from build123d import *

# Parameters (mm, degrees)
SKETCH1_W                = 50
SKETCH1_H                = 25
SKETCH1_R                = 1.3
SKETCH1_R_2              = 4.5
BOSS_EXTRUDE1_DEPTH      = 2.5
SKETCH2_W                = 50
SKETCH2_H                = 12
BOSS_EXTRUDE2_DEPTH      = 3
SKETCH3_W                = 50
SKETCH3_H                = 28
BOSS_EXTRUDE3_DEPTH      = 3
SKETCH4_R                = 1.3
CUT_EXTRUDE1_DEPTH       = 16
SKETCH5_W                = 53
SKETCH5_H                = 32.5
SKETCH5_R                = 1.6
SKETCH5_W_2              = 42
SKETCH5_H_2              = 21.5
BOSS_EXTRUDE4_DEPTH      = 4
SKETCH7_R                = 8
CUT_EXTRUDE2_DEPTH       = 5
SKETCH8_W                = 24.55
SKETCH8_H                = 21.5
CUT_EXTRUDE3_DEPTH       = 3.8
BOSS_EXTRUDE6_DEPTH      = 22.95
BOSS_EXTRUDE7_DEPTH      = 2
SKETCH11_R               = 1.6
CUT_EXTRUDE4_DEPTH       = 1.2
SKETCH12_W               = 7
SKETCH12_H               = 21
SKETCH12_R               = 1.6
BOSS_EXTRUDE8_DEPTH      = 7.8
SKETCH13_W               = 0.7
SKETCH13_H               = 5
SKETCH13_H_2             = 4
CUT_EXTRUDE5_DEPTH       = 51
CUT_EXTRUDE5_DEPTH_BACK  = 25.95
SKETCH14_W               = 3
SKETCH14_H               = 4
SKETCH14_W_2             = 25
SKETCH14_H_2             = 5
CUT_EXTRUDE6_DEPTH       = 1
CUT_EXTRUDE6_DEPTH_BACK  = 75.95
SKETCH15_W               = 24.95
SKETCH15_H               = 3
CUT_EXTRUDE7_DEPTH       = 11
CUT_EXTRUDE7_DEPTH_BACK  = 6
SKETCH16_R               = 1.45
SKETCH16_W               = 6
SKETCH16_H               = 5.2
CUT_EXTRUDE8_DEPTH       = 1
CUT_EXTRUDE8_DEPTH_BACK  = 29
SKETCH18_R               = 1.5
CUT_EXTRUDE9_DEPTH       = 1
CUT_EXTRUDE9_DEPTH_BACK  = 16
SKETCH19_R               = 1.3
BOSS_EXTRUDE9_DEPTH      = 3
SKETCH20_R               = 1.5
CUT_EXTRUDE10_DEPTH      = 1
CUT_EXTRUDE10_DEPTH_BACK = 16


with BuildPart() as part:
    # Sketch1 → Boss-Extrude1 (new body, symmetric)
    with BuildSketch(Plane(origin=(0, 0, 0), x_dir=(1, 0, 0), z_dir=(0, 1, 0))):
        Rectangle(SKETCH1_W, SKETCH1_H)
        with Locations((-11.25, 0)):
            Circle(SKETCH1_R, mode=Mode.SUBTRACT)
        with Locations((11.25, 0)):
            Circle(SKETCH1_R_2, mode=Mode.SUBTRACT)
    extrude(amount=BOSS_EXTRUDE1_DEPTH, both=True)

    # Sketch2 → Boss-Extrude2 (add)
    with BuildSketch(Plane.XY.offset(12.5)):
        with Locations((0, 3.5)):
            Rectangle(SKETCH2_W, SKETCH2_H)
    extrude(amount=BOSS_EXTRUDE2_DEPTH)

    # Sketch3 → Boss-Extrude3 (add)
    with BuildSketch(Plane(origin=(0, 9.5, 0), x_dir=(1, 0, 0), z_dir=(0, 1, 0))):
        with Locations((0, -1.5)):
            Rectangle(SKETCH3_W, SKETCH3_H)
    extrude(amount=BOSS_EXTRUDE3_DEPTH)

    # Sketch4 → Cut-Extrude1 (cut, through all)
    with BuildSketch(Plane(origin=(0, 12.5, 0), x_dir=(1, 0, 0), z_dir=(0, 1, 0))):
        with Locations((11.25, 0)):
            Circle(SKETCH4_R)
        with Locations((-11.25, 0)):
            Circle(SKETCH4_R)
    extrude(amount=-CUT_EXTRUDE1_DEPTH, mode=Mode.SUBTRACT)

    # Sketch5 → Boss-Extrude4 (add)
    with BuildSketch(Plane.XZ.offset(2.5)):
        with Locations((21.45, -0.05)):
            Rectangle(SKETCH5_W, SKETCH5_H)
        with Locations((45.75, -5)):
            Circle(SKETCH5_R, mode=Mode.SUBTRACT)
        with Locations((45.75, 4.9)):
            Circle(SKETCH5_R, mode=Mode.SUBTRACT)
        with Locations((-2.85, 4.9)):
            Circle(SKETCH5_R, mode=Mode.SUBTRACT)
        with Locations((-2.85, -5)):
            Circle(SKETCH5_R, mode=Mode.SUBTRACT)
        with Locations((21.45, -0.05)):
            Rectangle(SKETCH5_W_2, SKETCH5_H_2, mode=Mode.SUBTRACT)
    extrude(amount=BOSS_EXTRUDE4_DEPTH)

    # Sketch7 → Cut-Extrude2 (cut)
    with BuildSketch(Plane.XZ.offset(2.5)):
        with Locations((11.25, 0)):
            Circle(SKETCH7_R)
    extrude(amount=-CUT_EXTRUDE2_DEPTH, mode=Mode.SUBTRACT)

    # Sketch8 → Cut-Extrude3 (cut)
    with BuildSketch(Plane.XZ.offset(2.5)):
        with Locations((12.725, -0.05)):
            Rectangle(SKETCH8_W, SKETCH8_H)
    extrude(amount=-CUT_EXTRUDE3_DEPTH, mode=Mode.SUBTRACT)

    # Sketch9 → Boss-Extrude6 (add)
    with BuildSketch(Plane(origin=(25, 0, 0), x_dir=(0, 0, -1), z_dir=(1, 0, 0))):
        Polygon((12.5, 2.5), (-16.2, 2.5), (-16.2, -2.5), (-10.7, -2.5), (-10.7, 1.3), (10.8, 1.3), (10.8, -2.5), (12.5, -2.5), align=None)
    extrude(amount=BOSS_EXTRUDE6_DEPTH)

    # Sketch10 → Boss-Extrude7 (add)
    with BuildSketch(Plane(origin=(47.95, 0, 0), x_dir=(0, 0, -1), z_dir=(1, 0, 0))):
        Polygon((16.3, -2.5), (12.5, -2.5), (12.5, 2.5), (-16.2, 2.5), (-16.2, -6.5), (16.3, -6.5), align=None)
    extrude(amount=BOSS_EXTRUDE7_DEPTH)

    # Sketch11 → Cut-Extrude4 (cut)
    with BuildSketch(Plane.XZ.offset(-1.3)):
        with Locations((-2.85, 4.9)):
            Circle(SKETCH11_R)
        with Locations((-2.85, -5)):
            Circle(SKETCH11_R)
        with Locations((45.75, 4.9)):
            Circle(SKETCH11_R)
        with Locations((45.75, -5)):
            Circle(SKETCH11_R)
    extrude(amount=-CUT_EXTRUDE4_DEPTH, mode=Mode.SUBTRACT)

    # Sketch12 → Boss-Extrude8 (add)
    with BuildSketch(Plane.XZ.offset(-1.3)):
        with Locations((46.45, 0.2)):
            Rectangle(SKETCH12_W, SKETCH12_H)
        with Locations((45.75, 4.9)):
            Circle(SKETCH12_R, mode=Mode.SUBTRACT)
        with Locations((45.75, -5)):
            Circle(SKETCH12_R, mode=Mode.SUBTRACT)
    extrude(amount=BOSS_EXTRUDE8_DEPTH)

    # Sketch13 → Cut-Extrude5 (cut, two sides)
    with BuildSketch(Plane.ZY.offset(-25)) as cut_extrude5_sk:
        with Locations((15.85, 0)):
            Rectangle(SKETCH13_W, SKETCH13_H)
        with Locations((15.85, -4.5)):
            Rectangle(SKETCH13_W, SKETCH13_H_2)
    extrude(amount=CUT_EXTRUDE5_DEPTH, mode=Mode.SUBTRACT)
    extrude(cut_extrude5_sk.sketch, amount=-CUT_EXTRUDE5_DEPTH_BACK, mode=Mode.SUBTRACT)

    # Sketch14 → Cut-Extrude6 (cut, two sides)
    with BuildSketch(Plane.ZY.offset(25)) as cut_extrude6_sk:
        with Locations((14, -4.5)):
            Rectangle(SKETCH14_W, SKETCH14_H)
        Polygon((-16.3, 2.5), (-16.3, -6.5), (12.5, -6.5), (12.5, -2.5), (-12.5, -2.5), (-12.5, 2.5), align=None)
        Rectangle(SKETCH14_W_2, SKETCH14_H_2)
    extrude(amount=CUT_EXTRUDE6_DEPTH, mode=Mode.SUBTRACT)
    extrude(cut_extrude6_sk.sketch, amount=-CUT_EXTRUDE6_DEPTH_BACK, mode=Mode.SUBTRACT)

    # Sketch15 → Cut-Extrude7 (cut, two sides)
    with BuildSketch(Plane(origin=(0, 2.5, 0), x_dir=(1, 0, 0), z_dir=(0, 1, 0))) as cut_extrude7_sk:
        with Locations((37.475, -14)):
            Rectangle(SKETCH15_W, SKETCH15_H)
    extrude(amount=CUT_EXTRUDE7_DEPTH, mode=Mode.SUBTRACT)
    extrude(cut_extrude7_sk.sketch, amount=-CUT_EXTRUDE7_DEPTH_BACK, mode=Mode.SUBTRACT)

    # Sketch16 → Cut-Extrude8 (cut, two sides)
    with BuildSketch(Plane.XY.offset(15.5)) as cut_extrude8_sk:
        with Locations((-11, 0)):
            Circle(SKETCH16_R)
        with Locations((11, 0)):
            Circle(SKETCH16_R)
        with Locations((-22, 0.1)):
            Rectangle(SKETCH16_W, SKETCH16_H)
        with Locations((0, 0.1)):
            Rectangle(SKETCH16_W, SKETCH16_H)
        with Locations((22, 0.1)):
            Rectangle(SKETCH16_W, SKETCH16_H)
    extrude(amount=CUT_EXTRUDE8_DEPTH, mode=Mode.SUBTRACT)
    extrude(cut_extrude8_sk.sketch, amount=-CUT_EXTRUDE8_DEPTH_BACK, mode=Mode.SUBTRACT)

    # Sketch18 → Cut-Extrude9 (cut, two sides)
    with BuildSketch(Plane(origin=(0, 12.5, 0), x_dir=(1, 0, 0), z_dir=(0, 1, 0))) as cut_extrude9_sk:
        with Locations((-8.7, 0)):
            Circle(SKETCH18_R)
    extrude(amount=CUT_EXTRUDE9_DEPTH, mode=Mode.SUBTRACT)
    extrude(cut_extrude9_sk.sketch, amount=-CUT_EXTRUDE9_DEPTH_BACK, mode=Mode.SUBTRACT)

    # Sketch19 → Boss-Extrude9 (add)
    with BuildSketch(Plane(origin=(0, 12.5, 0), x_dir=(1, 0, 0), z_dir=(0, 1, 0))):
        with BuildLine():
            ThreePointArc((-10.084803922, -0.57647038), (-10.2, 0), (-10.084803922, 0.57647038))
            ThreePointArc((-10.084803922, 0.57647038), (-12.55, 0), (-10.084803922, -0.57647038))
        make_face()
        with Locations((11.25, 0)):
            Circle(SKETCH19_R)
    extrude(amount=-BOSS_EXTRUDE9_DEPTH)

    # Sketch20 → Cut-Extrude10 (cut, two sides)
    with BuildSketch(Plane(origin=(0, 12.5, 0), x_dir=(1, 0, 0), z_dir=(0, 1, 0))) as cut_extrude10_sk:
        with Locations((13.8, 0)):
            Circle(SKETCH20_R)
    extrude(amount=CUT_EXTRUDE10_DEPTH, mode=Mode.SUBTRACT)
    extrude(cut_extrude10_sk.sketch, amount=-CUT_EXTRUDE10_DEPTH_BACK, mode=Mode.SUBTRACT)


solid = part.part
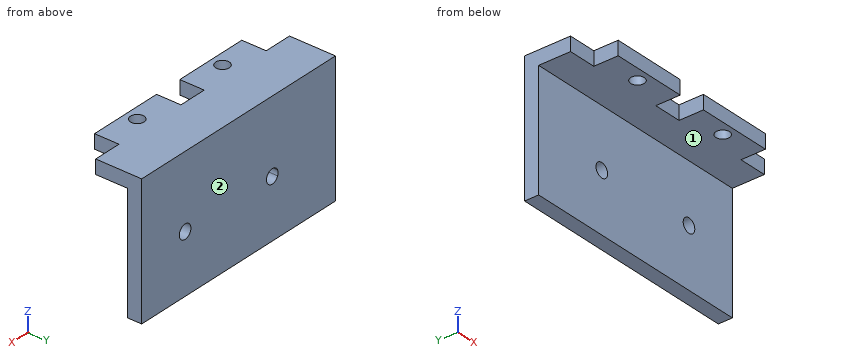
Source: CAD feature listing. Evaluate the final solid. Frame: model axes, mm. Face numbers are marked on the shaded views. A direction names the side the tool comes from. Coordinates: 2 decimals unless noted, no trailing zeros. Order: outer loops, then holes, each group sorted by start corner. A loop starts at its lowest first (then second) coordinate and runs counter-clockwise, first axis right, second up. Notation, with made-up numbers: M 58,51 L 74,51 A25 cw 74,63 Z; hole C -38.75,74.5 d9. An arc over 180 degrees is marked long. Write each question's results on one line, items separated by ' | '. Start each with the question number.
Item 1: Set-up query: the marked faces 1 and 2. Return all of +Z, -Z, +X, -X, +Y, -Y with unobstructed straight access to the full face (end or side cutting, diameter ignored); none if empty.
Item 2: Cut plane C-C (z = 0). Return loops of the section in (x, y).
Item 3: Cut plane A-A (x = -11). Return loops of the section in (y, z), and give its area (3 significant figures).
Item 4: First-contact query: pin 1 Ø2.5 at (x, z) = (0, 13.5) entering from -Y; pin 2 Ø3.5 at (y, z) = (0, 14) entering from +X; pin 3 Ø1.5 at (y, z) = (0.5, 13.5) entering from -X; pin 4 Ø4.5 at (x, y) = (11, 0) entering from +Z. Flat tips, straight axial feed; report the tip coordinate or a pass-through.
Item 5: Cut plane B-B (y = 0). Return loops of the section in (x, z), and give its area (3 significant figures).
Item 6: Cut plane D-D (x = -2.5). Return loops of the section in (y, z), and give its area (3 significant figures).
Item 7: Line query: probe 1 along Y at (x, z) = (-11, 14.85); probe 2 along Z at (x, y) = (8, -2); probe 3 along Y at (x, z) = (20, 13.25). Output: solid intervals per line, ascending.
Checked values:
1) face 1: -Z, +X, -X, -Y | face 2: +Z, -Z, +X, -X, +Y
2) outline: M -25,9.5 L -10.2,9.5 L -10.2,12.5 L -25,12.5 Z; M -7.2,9.5 L 12.3,9.5 L 12.3,12.5 L -7.2,12.5 Z; M 15.3,9.5 L 25,9.5 L 25,12.5 L 15.3,12.5 Z
3) outline: M -2.5,12.5 L -1.45,12.5 L -1.45,15.5 L -2.5,15.5 Z; M 1.45,12.5 L 9.5,12.5 L 9.5,-12.5 L 12.5,-12.5 L 12.5,15.5 L 1.45,15.5 Z | area: 111 mm2
4) pin 1: stops at y = 2.7 | pin 2: stops at x = 19 | pin 3: stops at x = -19 | pin 4: stops at z = 15.5
5) outline: M -19,12.5 L -12.45,12.5 L -12.45,15.5 L -19,15.5 Z; M -9.55,12.5 L -3,12.5 L -3,15.5 L -9.55,15.5 Z; M 3,12.5 L 9.55,12.5 L 9.55,15.5 L 3,15.5 Z; M 12.45,12.5 L 19,12.5 L 19,15.5 L 12.45,15.5 Z | area: 78.6 mm2
6) outline: M 2.7,12.5 L 9.5,12.5 L 9.5,-12.5 L 12.5,-12.5 L 12.5,15.5 L 2.7,15.5 Z | area: 104 mm2
7) probe 1: y = -2.5 to -1.45, 1.45 to 12.5 | probe 2: z = 12.5 to 15.5 | probe 3: y = 2.7 to 12.5
